Geometry check sheet. Reference: drawing and pictorial views, mm from the part's lowest x, y, z. Give positions to 0.01 mm unless a question says otherwise; leave off trailing zeros. Loops run counter-clockwise (first coordinate to the right, second up) from the corner with the lowest first, then second, coordinate; pieces in that order, holes last. Notation, with made-up numbers: (35.5, 80) -> (68.5, 80) arc R32 cw to (68.5, 112) -> close; hole circle Ø6 at (59, -39.5). An arc over 180 degrees is marked (long way). One line per item, written item: value. Start each with the question number.
(1) Sectioned sample at C-C, the plane y = 0.65. Record the cut outline in (x, z), then the cut area to 3 significant figures.
(2) Sectioned sample at D-D, the plane z = 4. Record the cut outline in (x, y), then the cut area to 3 significant figures.
(3) Scan lines: line 1 along Z through (x, y) = (29.75, 2.3); line 2 along Z through (x, y) = (42.5, 0.55); line 3 along X through (y, z) = (3.8, 19.25). Record each from-to range of solid material in increasing order. Write a range as from..to.
(4) Sectioned sample at B-B, the plane x = 5.75. Record the cut outline in (y, z), then the cut area to 3 significant figures.
(5) Gauge pin test, flat ends, axial feed: pin 1 Ø2.5 at (x, z) = (42.5, 5) entering from -Y; pin 2 Ø4.5 at (x, z) = (29.75, 20) entering from -Y. Record the tip position at first contact, or that the pin passes through.
(6) Sectioned sample at A-A, the plane x = 49.5. Record the cut outline in (y, z).
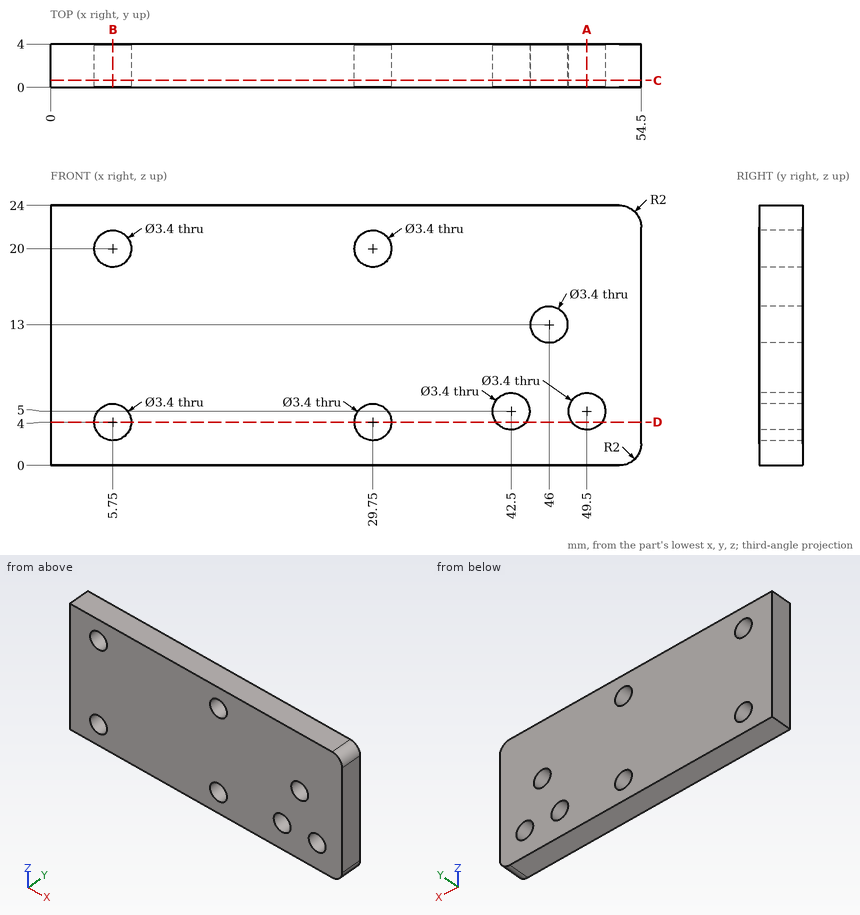
Calculated:
1. outline: (0, 0) -> (52.5, 0) arc R2 ccw to (54.5, 2) -> (54.5, 22) arc R2 ccw to (52.5, 24) -> (0, 24) -> close; hole circle Ø3.4 at (5.75, 4); hole circle Ø3.4 at (5.75, 20); hole circle Ø3.4 at (29.75, 4); hole circle Ø3.4 at (29.75, 20); hole circle Ø3.4 at (42.5, 5); hole circle Ø3.4 at (46, 13); hole circle Ø3.4 at (49.5, 5)
1. area: 1,240 mm2
2. outline: (0, 0) -> (4.05, 0) -> (4.05, 4) -> (0, 4) -> close; (7.45, 0) -> (28.05, 0) -> (28.05, 4) -> (7.45, 4) -> close; (31.45, 0) -> (41.13, 0) -> (41.13, 4) -> (31.45, 4) -> close; (43.87, 0) -> (48.13, 0) -> (48.13, 4) -> (43.87, 4) -> close; (50.87, 0) -> (54.5, 0) -> (54.5, 4) -> (50.87, 4) -> close
2. area: 169 mm2
3. line 1: z = 0..2.3, 5.7..18.3, 21.7..24
3. line 2: z = 0..3.3, 6.7..24
3. line 3: x = 0..4.22, 7.28..28.22, 31.28..54.5
4. outline: (0, 0) -> (4, 0) -> (4, 2.3) -> (0, 2.3) -> close; (0, 5.7) -> (4, 5.7) -> (4, 18.3) -> (0, 18.3) -> close; (0, 21.7) -> (4, 21.7) -> (4, 24) -> (0, 24) -> close
4. area: 68.8 mm2
5. pin 1: passes through
5. pin 2: stops at y = 0
6. outline: (0, 0) -> (4, 0) -> (4, 3.3) -> (0, 3.3) -> close; (0, 6.7) -> (4, 6.7) -> (4, 24) -> (0, 24) -> close
